from build123d import *

# Parameters (mm, degrees)
EXTRUDE_THIN1_DEPTH = 476.25
FILLET1_R           = 1.27


with BuildPart() as part:
    # Sketch1 → Extrude-Thin1 (new body)
    with BuildSketch(Plane.XY):
        with BuildLine():
            Line((-17.4625, 0), (-23.8125, 0))
            Line((-23.8125, 0), (-23.8125, -3.175))
            ThreePointArc((-23.8125, -3.175), (-19.4649522, -4.471511039), (-16.537661084, -7.9375))
            ThreePointArc((-16.537661084, -7.9375), (-8.60836669, -4.370835686), (0, -3.149841478))
            Line((0, -3.149841478), (0, -1.879841478))
            ThreePointArc((0, -1.879841478), (-8.305471157, -2.968488199), (-16.049802005, -6.160876419))
            ThreePointArc((-16.049802005, -6.160876419), (-18.838548597, -3.364089602), (-22.5425, -1.993006799))
            Line((-22.5425, -1.993006799), (-22.5425, -1.27))
            Line((-22.5425, -1.27), (-17.4625, -1.27))
            Line((-17.4625, -1.27), (-17.4625, 0))
        make_face()
    extrude(amount=-EXTRUDE_THIN1_DEPTH)

    # Mirror1: part across plane


with BuildPart() as part_1:
    add(part.part)
    add(part.part.mirror(Plane(origin=(0, -1.879841478, -476.25), x_dir=(0, 0, 1), z_dir=(-1, 0, 0))))

    # Fillet1
    fillet1_edges = [part_1.edges().sort_by_distance(p)[0] for p in [
        (-16.537661084, -7.9375, -238.125),
        (-23.8125, -3.175, -238.125),
        (-23.8125, 0, -238.125),
        (16.537661084, -7.9375, -238.125),
        (23.8125, -3.175, -238.125),
        (23.8125, 0, -238.125),
    ]]
    fillet(fillet1_edges, radius=FILLET1_R)


solid = part_1.part
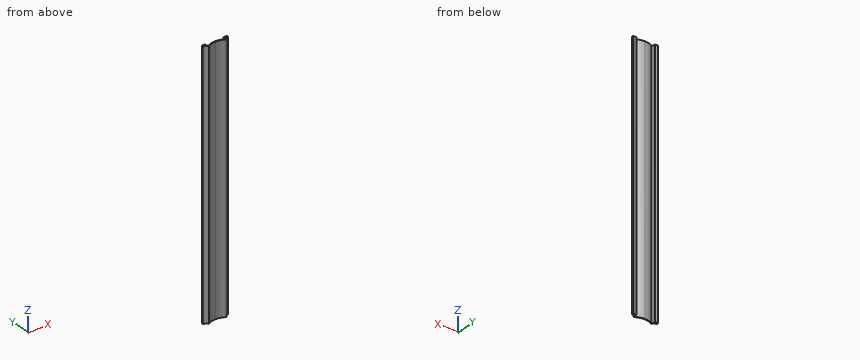
Model file for the job. Use its own axes, mm. Round coordinates to 2 decimals unless told otherwise and drop trailing zeros. Order: outer loops, then holes, each group sorted by start corner. A loop starts at its lowest first (then second) coordinate and runs counter-clockwise, first axis right, second up. Notation, with made-up numbers: M 43.5,23.25 L 73.5,23.25 A18 ccw 73.5,55.25 Z; hole C -33,45 d1. An arc over 180 degrees is marked long. Write each question's results on one line, items separated by ' | '. Start each with the question number.
(1) Drop flat-ended pins along their axis: pin 1 (1 mm diameter, centred on y = -5.5, z = -213, fed in from -X); pin 2 (5.5 mm diameter, centred on x = 20, z = -348.5, fed in from -Y); pin 3 (1 mm diameter, centred on y = -0.5, z = -243.5, fed in from -X). Give the stop position or say it passes through.
(2) Saw through at B-B, the plane x = -5.5. Give the cut face in (y, z), then the cut area to 3 significant figures.
(3) Probe probe 1 along X at (y, z) = (-5.5, -343); probe 2 along Y at (x, z) = (-17.5, -97.5); probe 3 along X at (y, z) = (-0.5, -313). List the from-to ranges inside material, lowest first. Write a range as from..to.
(4) Saw through at A-A, the plane y = -4.5. Give the cut face in (x, z).
Established:
1) pin 1: stops at x = -18.75 | pin 2: stops at y = -6.65 | pin 3: stops at x = -23.78
2) outline: M -3.64,-476.25 L -2.35,-476.25 L -2.35,0 L -3.64,0 Z | area: 614 mm^2
3) probe 1: x = -18.2..-16.51, -14.84..-11.83, 11.83..14.84, 16.51..18.2 | probe 2: y = -6.3..-4.41, -1.27..0 | probe 3: x = -23.55..-17.46, 17.46..23.55
4) outline: M -19.42,-476.25 L -17.41,-476.25 L -17.41,0 L -19.42,0 Z; M -12.73,-476.25 L -9.04,-476.25 L -9.04,0 L -12.73,0 Z; M 9.04,-476.25 L 12.73,-476.25 L 12.73,0 L 9.04,0 Z; M 17.41,-476.25 L 19.42,-476.25 L 19.42,0 L 17.41,0 Z
